Check sheet for the modelled part. Datum: model origin and axes. Units: mm. Face numbers are marked on the shaded views. A direction names the side the tool comes from. Round coordinates to 2 decimals unless told otherwise and drop trailing zeros. Write each loop counter-clockwise with the first axis right and the second up, starting at its lowest first coordinate (ties: lowest second). Pieces come first, ordered by that corner, then holes. Notation, with made-up numbers: (32.25, 10.5) -> (37.25, 10.5) arc R17 ccw to (37.25, 39.5) -> close; hole circle Ø1 at (82.25, 52). An arc over 180 degrees is marked (long way). One line per item, written item: value.
from build123d import *

# Parameters (mm, degrees)
BOSS_EXTRUDE1_DEPTH = 1.5
SKETCH2_W           = 58.49874
SKETCH2_H           = 5.00126
BOSS_EXTRUDE2_DEPTH = 8.5
SKETCH3_W           = 10
SKETCH3_H           = 7.5
SKETCH3_H_2         = 9
BOSS_EXTRUDE3_DEPTH = 9
SKETCH4_R           = 4
BOSS_EXTRUDE4_DEPTH = 7
FILLET1_R           = 2.54
FILLET2_R           = 1.27


with BuildPart() as part:
    # Sketch1 → Boss-Extrude1 (new body)
    with BuildSketch(Plane(origin=(0, 0, 0), x_dir=(1, 0, 0), z_dir=(0, 1, 0))):
        Polygon((-29.009375, 25.8421875), (29.990625, 25.8421875), (29.990625, 11.3421875), (27.990625, 11.3421875), (27.990625, -8.6578125), (29.990625, -8.6578125), (29.990625, -23.1578125), (-29.009375, -23.1578125), (-29.009375, -14.6578125), (-40.009375, -14.6578125), (-40.009375, 17.3421875), (-29.009375, 17.3421875), align=None)
    extrude(amount=BOSS_EXTRUDE1_DEPTH)

    # Sketch2 → Boss-Extrude2 (add)
    with BuildSketch(Plane(origin=(0, 1.5, 0), x_dir=(1, 0, 0), z_dir=(0, 1, 0))):
        with Locations((0.489995, -20.1571825)):
            Rectangle(SKETCH2_W, SKETCH2_H)
        with Locations((0.489995, 22.8415575)):
            Rectangle(SKETCH2_W, SKETCH2_H)
    extrude(amount=BOSS_EXTRUDE2_DEPTH)

    # Sketch3 → Boss-Extrude3 (add)
    with BuildSketch(Plane(origin=(0, 1.5, 0), x_dir=(1, 0, 0), z_dir=(0, 1, 0))):
        with Locations((-34.509375, 10.0921875)):
            Rectangle(SKETCH3_W, SKETCH3_H)
        with Locations((-34.509375, 1.3421875)):
            Rectangle(SKETCH3_W, SKETCH3_H_2)
        with Locations((-34.509375, -7.4078125)):
            Rectangle(SKETCH3_W, SKETCH3_H)
    extrude(amount=BOSS_EXTRUDE3_DEPTH)

    # Sketch4 → Boss-Extrude4 (add)
    with BuildSketch(Plane(origin=(0, 1.5, 0), x_dir=(1, 0, 0), z_dir=(0, 1, 0))):
        with Locations(Location((-24.009375, 15.3409275, 0), (0, 0, 90))):
            Circle(SKETCH4_R)
        with Locations(Location((-24.009375, -12.6565525, 0), (0, 0, 90))):
            Circle(SKETCH4_R)
    extrude(amount=BOSS_EXTRUDE4_DEPTH)

    # Fillet1
    fillet1_edges = [part.edges().sort_by_distance(p)[0] for p in [
        (-29.009375, 0.75, 14.6578125),
        (-29.009375, 0.75, -17.3421875),
    ]]
    fillet(fillet1_edges, radius=FILLET1_R)

    # Fillet2
    fillet2_edges = [part.edges().sort_by_distance(p)[0] for p in [
        (27.990625, 0.75, -11.3421875),
        (27.990625, 0.75, 8.6578125),
    ]]
    fillet(fillet2_edges, radius=FILLET2_R)


solid = part.part
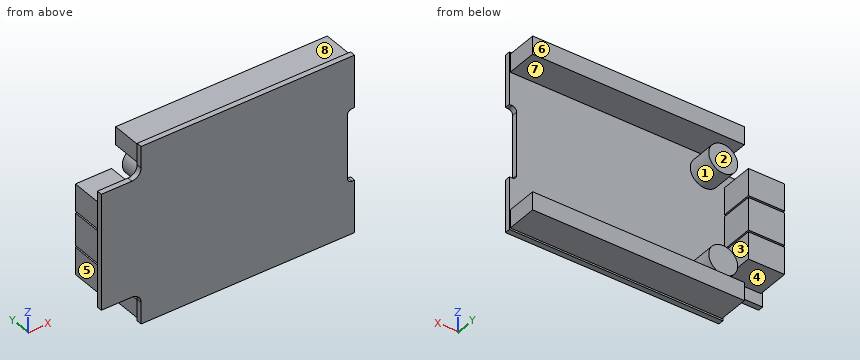
Item 1: Depth check by flat-ended pin: pin 1 (12 mm diameter, centred on x = -8.5, z = -6.5, fed in from +Y); pin 2 (4.5 mm diameter, centred on x = -34.5, y = 7, fed in from -Z); pin 3 (4 mm diameter, centred on y = 9, z = 15, fed in from +X). Enter the tip coordinate at first touch or a pass-through.
Result set:
pin 1: y = 1.5
pin 2: z = -13.84
pin 3: x = -20.03
Item 2: Sectioned sample at A-A (y = 5.75). Enter the section's corners in (x, z), then the cut area to 3 significant figures.
Result set:
outline: (-39.51, -13.84) -> (-29.51, -13.84) -> (-29.51, -6.34) -> (-39.51, -6.34) -> close; (-39.51, -5.84) -> (-29.51, -5.84) -> (-29.51, 3.16) -> (-39.51, 3.16) -> close; (-39.51, 3.66) -> (-29.51, 3.66) -> (-29.51, 11.16) -> (-39.51, 11.16) -> close; (-28.76, -25.34) -> (29.74, -25.34) -> (29.74, -20.34) -> (-28.76, -20.34) -> close; (-28.76, 17.66) -> (29.74, 17.66) -> (29.74, 22.66) -> (-28.76, 22.66) -> close; circle Ø8 at (-24.01, -15.34); circle Ø8 at (-24.01, 12.66)
area: 926 mm^2
Item 3: Release check for a two-part mould opening along Z. For the marked faces 6, 7 and 8 record: pulls with the +Z half, pulls with the -Z half, needs draft (parallel to the pull), parting line crosses it, or undercut.
Result set:
face 6: needs draft
face 7: undercut
face 8: pulls with the +Z half
Item 4: Sectioned sample at B-B (x = 7.5). Enter the section's corners in (y, z).
Result set:
outline: (0, -25.84) -> (1.5, -25.84) -> (1.5, -25.34) -> (10, -25.34) -> (10, -20.34) -> (1.5, -20.34) -> (1.5, 17.66) -> (10, 17.66) -> (10, 22.66) -> (1.5, 22.66) -> (1.5, 23.16) -> (0, 23.16) -> close
Item 5: Sectioned sample at D-D (z = 6). Enter the section's corners in (x, y), then the cut area to 3 significant figures.
Result set:
outline: (-40.01, 0) -> (27.99, 0) -> (27.99, 1.5) -> (-29.51, 1.5) -> (-29.51, 10.5) -> (-39.51, 10.5) -> (-39.51, 1.5) -> (-40.01, 1.5) -> close
area: 192 mm^2
Item 6: Tool access check on the marked faces 1, 2, 3, 4 and 5. Record the directions out of +Z, -Z, +X, -X, +Y, -Y that give a thin tool (end or side, any length) a straight path to the whole face; none if there is none.
Result set:
face 1: +Y
face 2: +X, +Y
face 3: +Z, -Z, +Y
face 4: -Z, -X, +Y
face 5: +Z, -Z, -X, +Y
Item 7: Sectioned sample at C-C (z = 19). Enter the section's corners in (x, y).
Result set:
outline: (-29.01, 0) -> (29.99, 0) -> (29.99, 1.5) -> (29.74, 1.5) -> (29.74, 10) -> (-28.76, 10) -> (-28.76, 1.5) -> (-29.01, 1.5) -> close
Item 8: Material ranges on line 1 along Z through (x, y) = (-32.5, 3.25); line 2 along Z through (x, y) = (16.5, 8.25); line 3 along Y through (x, z) = (-18.5, 10), recorded low to high.
Result set:
line 1: -13.84 to -6.34, -5.84 to 3.16, 3.66 to 11.16
line 2: -25.34 to -20.34, 17.66 to 22.66
line 3: 0 to 1.5
